Build history of the part. All positions in model axes, mm. Face numbers are marked on the shaded views. A direction names the side the tool comes from. Round coordinates to 2 decimals unless told otherwise and drop trailing zeros. Loops run counter-clockwise (first coordinate to the right, second up) from the corner with the lowest first, then second, coordinate; pieces in that order, holes last. Notation, with made-up numbers: (59.5, 4.25) -> (110.5, 4.25) arc R16 cw to (110.5, 27.25) -> close; hole circle Ø11 at (24, -34). An arc over 180 degrees is marked (long way). Put each result on its own line as item: value. Start each with the question number.
Item 1: Pull direction Y, two halves, no side cores. Call the marked faces 4, 5 and 6: +Y half, -Y half, draft (parallel to the pull), parting line (faces both ways), or undercut.
Item 2: Flat gauge pins, fed straight in: pin 1 Ø1.5 at (x, z) = (-2, 8.5) entering from +Y; pin 2 Ø4 at (x, z) = (1.5, 5.5) entering from +Y; pin 3 Ø3 at (y, z) = (-3, 11) entering from -X. Where does each tip first touch, or does it go through?
Item 3: Drill centre lines: probe 1 along Z at (x, y) = (1, 3.25); probe 2 along Z at (x, y) = (0, -1.25); probe 3 along X at (y, z) = (-1.5, 7.25). Where is each one in solid material? Low to high. Write a range as [from, to].
Item 4: Cut at C-C, the plane z = 6.5. List the corners of the cut face in (x, y).
Item 5: Cut at A-A, the plane z = 11.25. List the corners of the cut face in (x, y).
Item 6: Tool access for the marked faces 1, 2 and 3: list every direction of +Z, -Z, +X, -X, +Y, -Y with a clear straight run to the whole face (end or side of a thin tool).
Item 7: Cut at B-B, the plane x = 0. List the corners of the cut face in (y, z), plus the area to 3 significant figures.
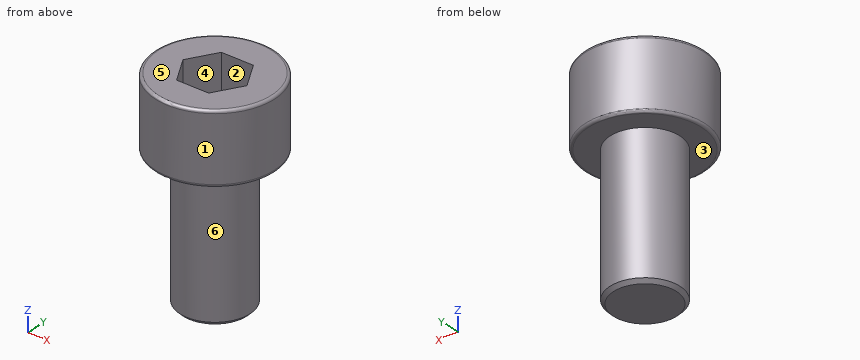
```python
from build123d import *

# Parameters (mm, degrees)
SKETCH1_R           = 4.25
BOSS_EXTRUDE1_DEPTH = 5
SKETCH2_R           = 2.5
BOSS_EXTRUDE2_DEPTH = 10
CUT_EXTRUDE1_DEPTH  = 4
CHAMFER1_SIZE       = 0.25
FILLET1_R           = 0.2


with BuildPart() as part:
    # Sketch1 → Boss-Extrude1 (new body)
    with BuildSketch(Plane.XY.offset(15)):
        with Locations(Location((0, 0, 0), (0, 0, 180))):
            Circle(SKETCH1_R)
    extrude(amount=-BOSS_EXTRUDE1_DEPTH)

    # Sketch2 → Boss-Extrude2 (add)
    with BuildSketch(Plane(origin=(0, 0, 10), x_dir=(-1, 0, 0), z_dir=(0, 0, -1))):
        Circle(SKETCH2_R)
    extrude(amount=BOSS_EXTRUDE2_DEPTH)

    # Sketch3 → Cut-Extrude1 (cut)
    with BuildSketch(Plane.XY.offset(15)):
        Polygon((-2.309401077, 0), (-1.154700538, -2), (1.154700538, -2), (2.309401077, 0), (1.154700538, 2), (-1.154700538, 2), align=None)
    extrude(amount=-CUT_EXTRUDE1_DEPTH, mode=Mode.SUBTRACT)

    # Chamfer1
    chamfer1_edges = [part.edges().sort_by_distance(p)[0] for p in [
        (2.5, 0, 0),
    ]]
    chamfer(chamfer1_edges, length=CHAMFER1_SIZE)

    # Fillet1
    fillet1_edges = [part.edges().sort_by_distance(p)[0] for p in [
        (4.25, 0, 15),
        (4.25, 0, 10),
    ]]
    fillet(fillet1_edges, radius=FILLET1_R)


solid = part.part
```
Reply:
1. face 4: undercut
1. face 5: draft
1. face 6: parting line
2. pin 1: stops at y = 2.17
2. pin 2: stops at y = 2.5
2. pin 3: stops at x = -3.98
3. probe 1: z = [10, 15]
3. probe 2: z = [0, 11]
3. probe 3: x = [-2, 2]
4. outline: circle Ø5 at (0, 0)
5. outline: circle Ø8.5 at (0, 0); hole (-2.31, 0) -> (-1.15, -2) -> (1.15, -2) -> (2.31, 0) -> (1.15, 2) -> (-1.15, 2) -> close
6. face 1: +Z, -Z
6. face 2: +Z
6. face 3: -Z
7. outline: (-4.25, 10.2) arc R0.2 ccw to (-4.05, 10) -> (-2.5, 10) -> (-2.5, 0.25) -> (-2.25, 0) -> (2.25, 0) -> (2.5, 0.25) -> (2.5, 10) -> (4.05, 10) arc R0.2 ccw to (4.25, 10.2) -> (4.25, 14.8) arc R0.2 ccw to (4.05, 15) -> (2, 15) -> (2, 11) -> (-2, 11) -> (-2, 15) -> (-4.05, 15) arc R0.2 ccw to (-4.25, 14.8) -> close
7. area: 76.4 mm^2
